```python
from build123d import *

# Parameters (mm, degrees)
F1_DEPTH = 15
F2_R     = 2.5
F3_DEPTH = 125.001
F4_R     = 7.49999
F5_R     = 5


# Not quite as in the source:
# - a fillet or chamfer is up to 0.001 mm smaller than in the source, because OpenCascade refuses the exact size


with BuildPart() as f1:
    # F0 (on Front) → F1 (new body)
    with BuildSketch(Plane.XZ):
        Polygon((-62.5, 23.75), (-62.5, -41.25), (62.5, -41.25), (62.5, 23.75), (62.5, 41.25), (52.5, 41.25), (52.5, 23.75), (-52.5, 23.75), (-52.5, 41.25), (-62.5, 41.25), align=None)
    extrude(amount=F1_DEPTH)

    # F2 (on face) → F3 (cut, through all)
    with BuildSketch(Plane.YZ.offset(62.5)):
        with Locations((-7.5, 33.75)):
            Circle(F2_R)
    extrude(amount=-F3_DEPTH, mode=Mode.SUBTRACT)

    # F4 (radius 7.5 in the source; OpenCascade refuses exactly that, so slightly less here)
    f4_edges = [f1.edges().sort_by_distance(p)[0] for p in [
        (57.5, 0, 41.25),
        (57.5, -15, 41.25),
        (-57.5, -15, 41.25),
        (-57.5, 0, 41.25),
    ]]
    fillet(f4_edges, radius=F4_R)

    # F5
    f5_edges = [f1.edges().sort_by_distance(p)[0] for p in [
        (0, 0, -41.25),
    ]]
    fillet(f5_edges, radius=F5_R)


solid = f1.part
```
CAD build for the part. Positions are in the model's coordinates, mm. A direction names the side the tool comes from. Round coordinates to 2 decimals unless told otherwise and drop trailing zeros. Write each loop counter-clockwise with the first axis right and the second up, starting at its lowest first coordinate (ties: lowest second). Pieces come first, ordered by that corner, then holes. Notation, with made-up numbers: M 51.5,-37.5 L 76.5,-37.5 A21 ccw 76.5,-15.5 Z; hole C -33.75,82.25 d6. An arc over 180 degrees is marked long. One line per question, with ' | ' between items.
1. Pin check, flat tips, straight feed: pin 1 Ø6 at (x, y) = (8.5, -2.5) entering from -Z; pin 2 Ø2 at (x, y) = (26.5, -11) entering from +Z. Stop position of each tip, or through.
Working result:
pin 1: z = -41.25 | pin 2: z = 23.75
2. Which spindle directions (+Z, -Z, +X, -X, +Y, -Y) get a long thin tool onto all of the face, cutting with end or side? Do faces 5 (the flat face through (-52.5, -7, 30)), 6 (the cylindrical face through (-57.57, -12.861, 38.995)). Say none if no direction does.
Working result:
face 5: +Z, +Y, -Y | face 6: +Z, +X, -X, -Y
3. Cut at B-B on x = 22. Write the cut outline in (y, z).
Working result:
outline: M -15,-41.25 L -5,-41.25 A5 ccw 0,-36.25 L 0,23.75 L -15,23.75 Z
4. Mould opens along X. For faces 1 (the flat face through (-1, -10, -41.25)), 2 (the flat face through (1, -7, 23.75)), 3 (the flat face through (52.5, -7, 31)), 4 (the flat face through (-62.5, -7, 1)) say: pulls with the +X half, pulls with the -X half, needs draft (parallel to the pull), parting line crosses it, or undercut.
Working result:
face 1: needs draft | face 2: undercut | face 3: undercut | face 4: pulls with the -X half
5. Probe L1, parallel to Z at x = 59.5, y = -7.5; L2, parallel to X at y = -9.75, z = 26; L3, parallel to Z at x = 35, y = -14. List the from-to ranges inside material, lowest first. Write a range as from..to.
Working result:
L1: -41.25..31.25, 36.25..41.25 | L2: -62.5..-52.5, 52.5..62.5 | L3: -41.25..23.75
6. Cut at A-A on y = -12. Write the cut outline in (x, z).
Working result:
outline: M -62.5,-41.25 L 62.5,-41.25 L 62.5,39.75 L 52.5,39.75 L 52.5,23.75 L -52.5,23.75 L -52.5,39.75 L -62.5,39.75 Z
